from build123d import *

# Parameters (mm, degrees)
F0_W     = 10
F0_H     = 10
F1_DEPTH = 25
F3_DEPTH = 5
F5_DEPTH = 10


with BuildPart() as f1:
    # F0 (on Top) → F1 (new body, symmetric)
    with BuildSketch(Plane.XY):
        Rectangle(F0_W, F0_H)
    extrude(amount=F1_DEPTH, both=True)

    # F2 (on face) → F3 (join)
    with BuildSketch(Plane(origin=(0, 0, -25), x_dir=(1, 0, 0), z_dir=(0, 0, -1))):
        with BuildLine():
            ThreePointArc((0, -5), (3.5355339059, -3.5355339059), (5, 0))
            ThreePointArc((5, 0), (3.5355339059, 3.5355339059), (0, 5))
            ThreePointArc((0, 5), (-3.5355339059, 3.5355339059), (-5, 0))
            ThreePointArc((-5, 0), (-3.5355339059, -3.5355339059), (0, -5))
        make_face()
    extrude(amount=F3_DEPTH)

    # F4 (on face) → F5 (join)
    with BuildSketch(Plane.XY.offset(25)):
        with BuildLine():
            ThreePointArc((0, -5), (3.5355339059, -3.5355339059), (5, 0))
            ThreePointArc((5, 0), (3.5355339059, 3.5355339059), (0, 5))
            ThreePointArc((0, 5), (-3.5355339059, 3.5355339059), (-5, 0))
            ThreePointArc((-5, 0), (-3.5355339059, -3.5355339059), (0, -5))
        make_face()
    extrude(amount=F5_DEPTH)


solid = f1.part
The listing builds one solid part. Answer for the finished solid, in the listing's coordinates (mm). A direction names the side the tool comes from. Give positions to 0.01 mm unless a question says otherwise; leave off trailing zeros. Write each loop counter-clockwise with the first axis right and the second up, starting at its lowest first coordinate (ties: lowest second). Pieces come first, ordered by that corner, then holes.
Item 1: Which of the six approach directions +Z, -Z, +X, -X, +Y, -Y give full straight-line access (tool end or side, diameter ignored) to faces 1 (the flat face through (4, -4, -25)), 2 (the flat face through (-4, -4, 25)), 3 (the flat face through (4, -4, 25))?
Item 2: Section B-B, the plane y = 2.5 is taken. Write down the section's boundary in (x, z), plus the area to 3 significant figures.
Item 3: Section A-A, the plane x = 3 is taken. Write down the section's boundary in (y, z), plus the area to 3 significant figures.
Item 4: Find the intervals of material crossed by line 1 along Z through (x, y) = (4.5, 4.5); line 2 along Y through (x, z) = (-0.75, 31.5); line 3 along Y through (x, z) = (1.5, 28), in increasing order.
Completed:
1. face 1: -Z, +X, -Y
1. face 2: +Z, -X, -Y
1. face 3: +Z, +X, -Y
2. outline: (-5, -25) - (-4.33, -25) - (-4.33, -30) - (4.33, -30) - (4.33, -25) - (5, -25) - (5, 25) - (4.33, 25) - (4.33, 35) - (-4.33, 35) - (-4.33, 25) - (-5, 25) - close
2. area: 630 mm2
3. outline: (-5, -25) - (-4, -25) - (-4, -30) - (4, -30) - (4, -25) - (5, -25) - (5, 25) - (4, 25) - (4, 35) - (-4, 35) - (-4, 25) - (-5, 25) - close
3. area: 620 mm2
4. line 1: z = -25 to 25
4. line 2: y = -4.94 to 4.94
4. line 3: y = -4.77 to 4.77
